Part model, mm, in its own coordinate system. A direction names the side the tool comes from. Coordinates: 2 decimals unless noted, no trailing zeros. Order: outer loops, then holes, each group sorted by start corner. A loop starts at its lowest first (then second) coordinate and runs counter-clockwise, first axis right, second up. Notation, with made-up numbers: (53, 79.5) - (87, 79.5) arc R23 ccw to (87, 92.5) - close; hole circle Ø4 at (-22, 58). An arc over 180 degrees is marked (long way). Use a Markdown table: item, result. Add a question column.
1) Drop flat-ended pins along their axis: P1, Ø2, axis at x = 12.5, z = -5, coming from the -Y side; P2, Ø5, axis at y = 4.5, z = -4.5, coming from the -X side; P3, Ø6, axis at x = 52.5, y = 3.5, coming from the -Z side; P4, Ø6, axis at x = 80, y = -4.5, coming from the -Z side. Give the stop position or say it passes through.
2) Saw through at A-A on z = 0. List the corners of the cut face in (x, y).
3) Wall check: L1, parallel to X at y = 1, z = 6.5; L2, parallel to Z at x = 16, y = 5.5; L3, parallel to Y at x = 100.5, z = -6. Give the ranges that are in metal, low to high. Write a range as [from, to].
4) Saw through at B-B on x = 66.5. List the corners of the cut face in (y, z).
5) Tool access for faces 1 (the face through (3.22, 4.65, 1.03)), 2 (the face through (106.35, 0, -5)), 3 (the face through (55.65, 3.219, 5.474)): list every direction of +Z, -Z, +X, -X, +Y, -Y with a clear straight run to the whole face (end or side of a thin tool).
6) Saw through at D-D on z = 6. List the corners of the cut face in (x, y).
7) Saw through at C-C on y = -3.25. List the corners of the cut face in (x, z).
```python
from build123d import *

# Parameters (mm, degrees)
SALIENTE_EXTRUIR1_DEPTH = 112.7
CROQUIS2_R              = 7.332348419
CROQUIS2_R_2            = 4.7625
CORTAR_EXTRUIR1_DEPTH   = 6.35
CORTAR_EXTRUIR2_START   = -6.35
CROQUIS3_R              = 7.332348419
CROQUIS3_R_2            = 4.7625
CORTAR_EXTRUIR2_DEPTH   = 6.35


with BuildPart() as part:
    # Croquis1 → Saliente-Extruir1 (new body)
    with BuildSketch(Plane(origin=(0, 0, 0), x_dir=(0, 0, -1), z_dir=(1, 0, 0))):
        Polygon((7.332348419, 0), (3.666174209, 6.35), (-3.666174209, 6.35), (-7.332348419, 0), (-3.666174209, -6.35), (3.666174209, -6.35), align=None)
    extrude(amount=SALIENTE_EXTRUIR1_DEPTH)

    # Croquis2 → Cortar-Extruir1 (cut)
    with BuildSketch(Plane(origin=(112.7, 0, 0), x_dir=(0, 0, -1), z_dir=(1, 0, 0))):
        Circle(CROQUIS2_R)
        Circle(CROQUIS2_R_2, mode=Mode.SUBTRACT)
    extrude(amount=-CORTAR_EXTRUIR1_DEPTH, mode=Mode.SUBTRACT)

    # Croquis3 → Cortar-Extruir2 (cut)
    with BuildSketch(Plane.ZY.offset(CORTAR_EXTRUIR2_START)):
        Circle(CROQUIS3_R)
        with Locations(Location((0, 0, 0), (0, 0, 180))):
            Circle(CROQUIS3_R_2, mode=Mode.SUBTRACT)
    extrude(amount=CORTAR_EXTRUIR2_DEPTH, mode=Mode.SUBTRACT)


solid = part.part
```
Results are:
| question | item | result |
|---|---|---|
| 1 | P1 | y = -5.77 |
| 1 | P2 | x = 0 |
| 1 | P3 | z = -7.04 |
| 1 | P4 | z = -6.47 |
| 2 | outline | (0, -4.76) - (6.35, -4.76) - (6.35, -6.35) - (106.35, -6.35) - (106.35, -4.76) - (112.7, -4.76) - (112.7, 4.76) - (106.35, 4.76) - (106.35, 6.35) - (6.35, 6.35) - (6.35, 4.76) - (0, 4.76) - close |
| 3 | L1 | [6.35, 106.35] |
| 3 | L2 | [-4.16, 4.16] |
| 3 | L3 | [-2.31, 2.31] |
| 4 | outline | (-6.35, -3.67) - (0, -7.33) - (6.35, -3.67) - (6.35, 3.67) - (0, 7.33) - (-6.35, 3.67) - close |
| 5 | face 1 | -X |
| 5 | face 2 | +X |
| 5 | face 3 | +Z, +X, -X, +Y |
| 6 | outline | (6.35, -2.31) - (106.35, -2.31) - (106.35, 2.31) - (6.35, 2.31) - close |
| 7 | outline | (0, -3.48) - (6.35, -3.48) - (6.35, -5.46) - (106.35, -5.46) - (106.35, -3.48) - (112.7, -3.48) - (112.7, 3.48) - (106.35, 3.48) - (106.35, 5.46) - (6.35, 5.46) - (6.35, 3.48) - (0, 3.48) - close |
